Read the model definition and answer for the solid it produces. Units are mm, in the model's axes. A direction names the side the tool comes from. Give positions to 0.01 mm unless a question says otherwise; leave off trailing zeros. Loops run counter-clockwise (first coordinate to the right, second up) from the corner with the lowest first, then second, coordinate; pieces in that order, holes last. Notation, with made-up numbers: (67, 52.25) - (80, 52.25) arc R16 ccw to (80, 69.25) - close; hole circle Ø4 at (-32, 27.5). An arc over 180 degrees is marked (long way). Write each question's results on one line, items separated by ' | '. Start each with the question number.
Q1. The part is cut by section B-B, the plane x = 181. Write down the section's boundary in (y, z).
Q2. Find the intervals of material crossed by line 1 (X direction, y = -15, z = 23); line 2 (Z direction, x = 113.5, y = -2); line 3 (X direction, y = -4.5, z = 27), in increasing order. Write a range as from..to.
Q3. Determine the mould class of faces 4 (the conical face through (424.875, -5.444, -17.288)), 5 (the flat face through (245, 9.9, 19.9)), 6 (the flat face through (298, 0, 15)) for opening direction Y: +Y half, -Y half, draft (parallel to the pull), parting line (faces both ways), or undercut.
Q4. Given pin 1 (1.7 mm diameter, centred on x = 74, z = 27.5, fed in from +Y); pin 2 (3.5 mm diameter, centred on x = 304.5, z = 17.5, fed in from -Y); pin 3 (5 mm diameter, centred on y = -23.5, z = -16.5, fed in from +X), each flat-ended and moving along its own axis, determine where each tip first touches the part or whether it passes through.
Q5. The part is cut by section C-C, the plane x = 89. Write down the section's boundary in (y, z), plus the area to 3 significant figures.
Q6. For faces 1 (the flat face through (40, -3.82, 22.34)), 2 (the cylindrical face through (209.51, 19.961, -10.382)), 3 (the flat face through (75, 0, 30)), determine the directions among +Z, -Z, +X, -X, +Y, -Y from which every point of the face is accessible in a straight line to the end or side of a thin tool.
```python
from build123d import *

# Parameters (mm, degrees)
CHAMFER1_SIZE       = 2
CUT_EXTRUDE2_DEPTH  = 5
CUT_EXTRUDE3_DEPTH  = 5
BOSS_EXTRUDE1_DEPTH = 10


with BuildPart() as part:
    # Sketch2 → Revolve1 (revolve)
    with BuildSketch(Plane(origin=(0, 0, 0), x_dir=(1, 0, 0), z_dir=(0, 1, 0))):
        Polygon((303.786030517, 20), (303.786030517, 0), (325, 0), (425, 0), (425, 20), (325, 20), align=None)
        Polygon((0, 22.5), (0, 0), (303.786030517, 0), (303.786030517, 20), (245, 20), (245, 22.5), (175, 22.5), (175, 30), (110, 30), (110, 25), (40, 25), (40, 22.5), align=None)
    revolve(axis=Axis((325, 0, 0), (-1, 0, 0)))

    # Chamfer1
    chamfer1_edges = [part.edges().sort_by_distance(p)[0] for p in [
        (425, 0, 20),
        (245, 0, 20),
    ]]
    chamfer(chamfer1_edges, length=CHAMFER1_SIZE)

    # Sketch4 → Cut-Extrude2 (cut)
    with BuildSketch(Plane.XY.offset(20)):
        with BuildLine():
            Line((257.357014361, -5), (345.693163579, -5))
            Line((345.693163579, -5), (345.693163579, 5))
            Line((345.693163579, 5), (257.357014361, 5))
            ThreePointArc((257.357014361, 5), (252.357014361, 0), (257.357014361, -5))
        make_face()
    extrude(amount=-CUT_EXTRUDE2_DEPTH, mode=Mode.SUBTRACT)

    # Sketch5 → Cut-Extrude3 (cut)
    with BuildSketch(Plane.XY.offset(25)):
        with BuildLine():
            Line((50, 5), (100, 5))
            ThreePointArc((100, 5), (105, 0), (100, -5))
            Line((100, -5), (50, -5))
            ThreePointArc((50, -5), (45, 0), (50, 5))
        make_face()
    extrude(amount=-CUT_EXTRUDE3_DEPTH, mode=Mode.SUBTRACT)

    # Sketch8 → Boss-Extrude1 (add)
    with BuildSketch(Plane.XY.offset(20)):
        with BuildLine():
            Line((100, 5), (50, 5))
            ThreePointArc((50, 5), (45, 0), (50, -5))
            Line((50, -5), (100, -5))
            ThreePointArc((100, -5), (105, 0), (100, 5))
        make_face()
    extrude(amount=BOSS_EXTRUDE1_DEPTH)


solid = part.part
```
Check sheet entries:
1) outline: circle Ø45 at (0, 0)
2) line 1: x = 110..175 | line 2: z = -29.93..29.93 | line 3: x = 47.82..102.18, 110..175
3) face 4: parting line | face 5: draft | face 6: undercut
4) pin 1: stops at y = 5 | pin 2: stops at y = -12.33 | pin 3: stops at x = 175
5) outline: (-5, 24.49) arc R25 ccw (long way) to (5, 24.49) - (5, 30) - (-5, 30) - close | area: 2,020 mm^2
6) face 1: -X | face 2: +X | face 3: +Z, +X, -X, +Y, -Y
